For this review, take the finished solid that the model builds, in its own axes (mm). Coordinates: 2 decimals unless noted, no trailing zeros. Write each loop counter-clockwise with the first axis right and the second up, starting at its lowest first coordinate (ties: lowest second). Pieces come first, ordered by that corner, then holes.
1) We need section A-A on z = 16. Write out the cut boundary in (x, y).
2) Insertion check: P1, Ø4, axis at x = -220.5, y = 89.5, coming from the -Z side; P2, Ø5, axis at y = 80.5, z = -6, coming from the +X side; P3, Ø2, axis at y = 120, z = -1.5, coming from the +X side. Each pin has a flat end and moves straight along its axis. Give the tip position at first contact, or say it passes through.
3) We need section C-C on z = 41.5. Write out the cut boundary in (x, y), then the cut area to 3 significant figures.
4) We need section B-B on z = 30. Write out the cut boundary in (x, y).
5) To check wall thickness, follow line 1 along X through (y, z) = (79.5, 27); line 2 along Z through (x, y) = (-183, 121); line 3 along Z through (x, y) = (-179, 119). State the ranges of each line that lie inside material, in increasing order.
6) Mouldability with a two-part tool opening along Y and no side actions: class faces 1 (the face through (-212.43, 104.29, -10.78)), 2 (the face through (-206.913, 95.952, -10.779)), 3 (the face through (-180.705, 119.181, 13.205)) as pulls with the +Y half, pulls with the -Y half, needs draft (parallel to the pull), parting line crosses it, or undercut.
Autodesk Inventor part; units mm, degrees
ref_plane "Work Plane1" through (-147.3677, -4.0754, 130.4495) normal (-0.5513437, 0.8342782, 0) x (0, 0, 1)
ref_plane "Work Plane2" through (-176.5966, 115.9868, 180.7146) normal (-0.5513437, 0.8342782, 0) x (0.1811695, 0.1197283, 0.9761366)
ref_plane "Work Plane3" through (-213.7676, 91.4218, -19.5622) normal (0.8143695, 0.5381868, -0.2171572) x (0.1811695, 0.1197283, 0.9761366)
ref_plane "Work Plane1" through (-147.3677, -4.0754, 130.4495) normal (-0.5513437, 0.8342782, 0) x (0, 0, 1)
ref_plane "Work Plane2" through (-176.5966, 115.9868, 180.7146) normal (-0.5513437, 0.8342782, 0) x (0.1811695, 0.1197283, 0.9761366)
sketch "Sketch2" plane through (-176.5966, 115.9868, 180.7146) normal (-0.5513437, 0.8342782, 0) x (0.1811695, 0.1197283, 0.9761366)
  arc A0 (82.4936, -40) -> (107.4936, -33.3012) centre (82.4936, 10) ccw
  line L0 (107.4936, -33.3012) -> (126.4432, -22.3607)
  arc A1 (132.9687, -23.7251) -> (126.4432, -22.3607) centre (128.9432, -26.6908) ccw
  arc A2 (132.9687, -23.7251) -> (132.9687, 23.7251) centre (165.173, 0) ccw
  arc A3 (126.4432, 22.3607) -> (132.9687, 23.7251) centre (128.9432, 26.6908) ccw
  line L1 (126.4432, 22.3607) -> (107.4936, 33.3012)
  arc A4 (107.4936, 33.3012) -> (82.4936, 40) centre (82.4936, -10) ccw
  line L2 (-82.4936, 40) -> (82.4936, 40)
  arc A5 (-82.4936, 40) -> (-107.4936, 33.3012) centre (-82.4936, -10) ccw
  line L3 (-107.4936, 33.3012) -> (-126.4432, 22.3607)
  arc A6 (-132.9687, 23.7251) -> (-126.4432, 22.3607) centre (-128.9432, 26.6908) ccw
  arc A7 (-132.9687, 23.7251) -> (-132.9687, -23.7251) centre (-165.173, 0) ccw
  arc A8 (-126.4432, -22.3607) -> (-132.9687, -23.7251) centre (-128.9432, -26.6908) ccw
  line L4 (-126.4432, -22.3607) -> (-107.4936, -33.3012)
  arc A9 (-107.4936, -33.3012) -> (-82.4936, -40) centre (-82.4936, 10) ccw
  line L5 (82.4936, -40) -> (-82.4936, -40)
  arc A10 (3.6764, 4.0958) -> (3.6764, -4.0958) centre (6.5442, 0) ccw
  line L6 (3.6764, -4.0958) -> (20.5406, -15.9042)
  arc A11 (17.6727, -25) -> (20.5406, -15.9042) centre (17.6727, -20) ccw
  line L7 (17.6727, -25) -> (-19.8928, -25)
  arc A12 (-22.7607, -24.0958) -> (-19.8928, -25) centre (-19.8928, -20) ccw
  line L8 (-22.7607, -24.0958) -> (-51.3236, -4.0958)
  arc A13 (-51.3236, 4.0958) -> (-51.3236, -4.0958) centre (-48.4558, 0) ccw
  line L9 (-51.3236, 4.0958) -> (-22.7607, 24.0958)
  arc A14 (-19.8928, 25) -> (-22.7607, 24.0958) centre (-19.8928, 20) ccw
  line L10 (-19.8928, 25) -> (17.6727, 25)
  arc A15 (20.5406, 15.9042) -> (17.6727, 25) centre (17.6727, 20) ccw
  line L11 (20.5406, 15.9042) -> (3.6764, 4.0958)
  line L12 (-50.2924, 21.3617) -> (-62.1293, 13.0734)
  arc A16 (-64.2764, 12.9796) -> (-62.1293, 13.0734) centre (-63.2764, 14.7117) ccw
  line L13 (-64.2764, 12.9796) -> (-78.6322, 21.2679)
  arc A17 (-77.6322, 25) -> (-78.6322, 21.2679) centre (-77.6322, 23) ccw
  line L14 (-77.6322, 25) -> (-51.4395, 25)
  arc A18 (-50.2924, 21.3617) -> (-51.4395, 25) centre (-51.4395, 23) ccw
  line L15 (-62.1293, -13.0734) -> (-50.2924, -21.3617)
  arc A19 (-51.4395, -25) -> (-50.2924, -21.3617) centre (-51.4395, -23) ccw
  line L16 (-51.4395, -25) -> (-77.6322, -25)
  arc A20 (-78.6322, -21.2679) -> (-77.6322, -25) centre (-77.6322, -23) ccw
  line L17 (-78.6322, -21.2679) -> (-64.2764, -12.9796)
  arc A21 (-62.1293, -13.0734) -> (-64.2764, -12.9796) centre (-63.2764, -14.7117) ccw
  line L18 (-102.673, -23.5566) -> (-119.3236, -13.9434)
  arc A22 (-121.8236, -9.6132) -> (-119.3236, -13.9434) centre (-116.8236, -9.6132) ccw
  line L19 (-121.8236, -9.6132) -> (-121.8236, 9.6132)
  arc A23 (-119.3236, 13.9434) -> (-121.8236, 9.6132) centre (-116.8236, 9.6132) ccw
  line L20 (-119.3236, 13.9434) -> (-102.673, 23.5566)
  arc A24 (-97.673, 23.5566) -> (-102.673, 23.5566) centre (-100.173, 19.2265) ccw
  line L21 (-97.673, 23.5566) -> (-81.0224, 13.9434)
  arc A25 (-78.5224, 9.6132) -> (-81.0224, 13.9434) centre (-83.5224, 9.6132) ccw
  line L22 (-78.5224, 9.6132) -> (-78.5224, -9.6132)
  arc A26 (-81.0224, -13.9434) -> (-78.5224, -9.6132) centre (-83.5224, -9.6132) ccw
  line L23 (-81.0224, -13.9434) -> (-97.673, -23.5566)
  arc A27 (-102.673, -23.5566) -> (-97.673, -23.5566) centre (-100.173, -19.2265) ccw
  line L24 (72.827, -25) -> (57.1072, -25)
  arc A28 (54.2393, -24.0958) -> (57.1072, -25) centre (57.1072, -20) ccw
  line L25 (54.2393, -24.0958) -> (25.6764, -4.0958)
  arc A29 (25.6764, 4.0958) -> (25.6764, -4.0958) centre (28.5442, 0) ccw
  line L26 (25.6764, 4.0958) -> (54.2393, 24.0958)
  arc A30 (57.1072, 25) -> (54.2393, 24.0958) centre (57.1072, 20) ccw
  line L27 (57.1072, 25) -> (72.827, 25)
  arc A31 (77.827, 20) -> (72.827, 25) centre (72.827, 20) ccw
  line L28 (77.827, 20) -> (77.827, -20)
  arc A32 (72.827, -25) -> (77.827, -20) centre (72.827, -20) ccw
  circle A33 centre (-165.173, 0) radius 11
  circle A34 centre (105.173, 0) radius 8
  line L29 (87.4451, -10.7279) -> (97.4451, -10.7279)
  arc A35 (97.4451, -14.7279) -> (97.4451, -10.7279) centre (97.4451, -12.7279) ccw
  line L30 (97.4451, -14.7279) -> (87.4451, -14.7279)
  arc A36 (87.4451, -10.7279) -> (87.4451, -14.7279) centre (87.4451, -12.7279) ccw
  line L31 (122.9009, -14.7279) -> (112.9009, -14.7279)
  arc A37 (112.9009, -10.7279) -> (112.9009, -14.7279) centre (112.9009, -12.7279) ccw
  line L32 (112.9009, -10.7279) -> (122.9009, -10.7279)
  arc A38 (122.9009, -14.7279) -> (122.9009, -10.7279) centre (122.9009, -12.7279) ccw
  line L33 (97.4451, 10.7279) -> (87.4451, 10.7279)
  arc A39 (87.4451, 14.7279) -> (87.4451, 10.7279) centre (87.4451, 12.7279) ccw
  line L34 (87.4451, 14.7279) -> (97.4451, 14.7279)
  arc A40 (97.4451, 10.7279) -> (97.4451, 14.7279) centre (97.4451, 12.7279) ccw
  line L35 (122.9009, 10.7279) -> (112.9009, 10.7279)
  arc A41 (112.9009, 14.7279) -> (112.9009, 10.7279) centre (112.9009, 12.7279) ccw
  line L36 (112.9009, 14.7279) -> (122.9009, 14.7279)
  arc A42 (122.9009, 10.7279) -> (122.9009, 14.7279) centre (122.9009, 12.7279) ccw
  line L37 (169.046, 1) -> (169.973, 1)
  line L38 (169.973, 1) -> (169.973, -1)
  line L39 (169.973, -1) -> (169.046, -1)
  arc A43 (169.046, 1) -> (169.046, -1) centre (165.173, 0) ccw
  circle A44 centre (158.2448, -4) radius 2
  circle A45 centre (172.1012, -4) radius 2
  circle A46 centre (165.173, 8) radius 2
  circle A47 centre (145.374, -19.799) radius 1.6
  circle A48 centre (165.173, -28) radius 1.6
  circle A49 centre (184.972, -19.799) radius 1.6
  circle A50 centre (193.173, 0) radius 1.6
  circle A51 centre (184.972, 19.799) radius 1.6
  circle A52 centre (165.173, 28) radius 1.6
  circle A53 centre (145.374, 19.799) radius 1.6
  circle A54 centre (137.173, 0) radius 1.6
  circle A55 centre (-165.173, -16.0004) radius 1.55
  circle A56 centre (-149.1726, 0) radius 1.55
  circle A57 centre (-165.173, 16.0004) radius 1.55
  circle A58 centre (-181.1734, 0) radius 1.55
  arc A59 (-141.0198, 17.7938) -> (-141.0198, -17.7938) centre (-165.173, 0) ccw
  arc A60 (-141.0198, 17.7938) -> (-121.4432, 13.7004) centre (-128.9432, 26.6908) ccw
  line L40 (-121.4432, 13.7004) -> (-102.4936, 24.641)
  arc A61 (-82.4936, 30) -> (-102.4936, 24.641) centre (-82.4936, -10) ccw
  line L41 (-82.4936, 30) -> (82.4936, 30)
  arc A62 (102.4936, 24.641) -> (82.4936, 30) centre (82.4936, -10) ccw
  line L42 (102.4936, 24.641) -> (121.4432, 13.7004)
  arc A63 (121.4432, 13.7004) -> (141.0198, 17.7938) centre (128.9432, 26.6908) ccw
  arc A64 (141.0198, -17.7938) -> (141.0198, 17.7938) centre (165.173, 0) ccw
  arc A65 (141.0198, -17.7938) -> (121.4432, -13.7004) centre (128.9432, -26.6908) ccw
  line L43 (121.4432, -13.7004) -> (102.4936, -24.641)
  arc A66 (82.4936, -30) -> (102.4936, -24.641) centre (82.4936, 10) ccw
  line L44 (82.4936, -30) -> (-82.4936, -30)
  arc A67 (-102.4936, -24.641) -> (-82.4936, -30) centre (-82.4936, 10) ccw
  line L45 (-102.4936, -24.641) -> (-121.4432, -13.7004)
  arc A68 (-121.4432, -13.7004) -> (-141.0198, -17.7938) centre (-128.9432, -26.6908) ccw
  arc A69 (-144.5699, -34.2857) -> (-149.7207, -25.7143) centre (-147.1453, -30) ccw
  line L46 (-205.173, 0) -> (-195.173, 0)
  arc A70 (-149.7207, 25.7143) -> (-144.5699, 34.2857) centre (-147.1453, 30) ccw
  point P0 (-158.2951, 120.6357)
  point P1 (-149.7207, 25.7143)
  point P2 (-144.5699, 34.2857)
  dimension "d4" = 10
  dimension "d5" = 30
extrude "Extrusion2" add sketch "Sketch2" along normal blind 10 contours A7 L46 A59 A69 | A7 A70 A59 L46
ref_plane "Work Plane3" through (-213.7676, 91.4218, -19.5622) normal (0.8143695, 0.5381868, -0.2171572) x (0.1811695, 0.1197283, 0.9761366)
sketch "Sketch3" plane through (-182.11, 124.3296, 180.7146) normal (-0.5513437, 0.8342782, 0) x (0.8143695, 0.5381868, -0.2171572)
  circle A0 centre (0, 200.673) radius 3.75
  circle A1 centre (35.5, 165.173) radius 3.75
  circle A2 centre (0, 129.673) radius 3.75
  circle A3 centre (-35.5, 165.173) radius 3.75
  circle A4 centre (-25.1023, 140.0707) radius 3.75
  circle A5 centre (25.1023, 140.0707) radius 3.75
  circle A6 centre (25.1023, 190.2753) radius 3.75
  circle A7 centre (-25.1023, 190.2753) radius 3.75
  circle A8 centre (0, 165.173) radius 40
  circle A9 centre (0, 165.173) radius 30.089
  point P0 (120.6357, 158.2951)
hole "Hole1" at (-218.4658, 100.3034, -15.1697) at (-196.1395, 115.058, -10.4712) at (-183.1242, 123.6594, 11.7741) at (-187.044, 121.0689, 38.5353) at (-205.6028, 108.8041, 54.136) at (-227.9291, 94.0495, 49.4376) at (-240.9444, 85.4481, 27.1923) at (-237.0246, 88.0386, 0.4311) direction (0.5513437, -0.8342782, 0) diameter 3 end through all
properties part number "spacer"
Result:
1. outline: (-245.28, 82.58) - (-239.77, 74.24) - (-231.38, 79.78) - (-236.89, 88.13) - close; (-187.18, 120.98) - (-181.66, 112.64) - (-173.28, 118.18) - (-178.79, 126.52) - close
2. P1: stops at z = -18.22
2. P2: stops at x = -226.51
2. P3: stops at x = -180.45
3. outline: (-239.9, 86.14) - (-234.38, 77.8) - (-223.9, 84.73) - (-229.41, 93.07) - close
3. area: 126 mm2
4. outline: (-244.23, 83.28) - (-238.72, 74.93) - (-229.96, 80.72) - (-235.47, 89.06) - close; (-188.48, 120.12) - (-182.97, 111.78) - (-174.32, 117.49) - (-179.84, 125.83) - close
5. line 1: x = -242.57 to -238.8, -235.23 to -231.81
5. line 2: z = -2.69 to 11.15, 12.4 to 35.57
5. line 3: z = 1.1 to 10.55, 12.99 to 34.99
6. face 1: pulls with the +Y half
6. face 2: pulls with the -Y half
6. face 3: undercut
